Could you check a few things on this model? Use its own coordinates, in mm. Coordinates: 2 decimals unless noted, no trailing zeros. Loops run counter-clockwise (first coordinate to the right, second up) from the corner with the lowest first, then second, coordinate; pieces in that order, holes last.
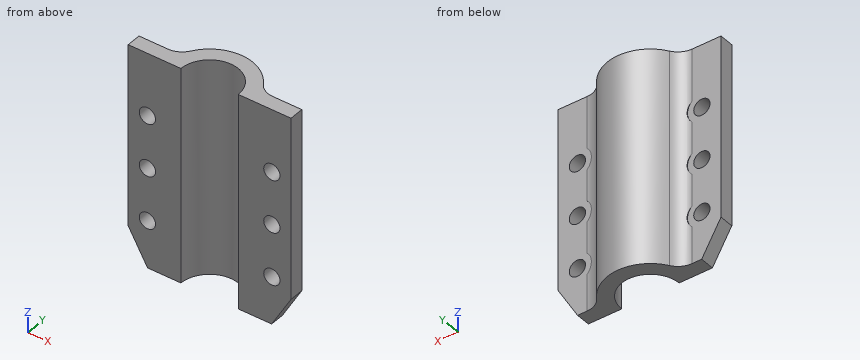
Autodesk Inventor part; units mm, degrees
ref_plane "Płaszczyzna konstrukcyjna1" through (0, 0, 50) normal (-1, 0, 0) x (0, 0, 1)
ref_plane "YZ Plane" through (0, 0, 0) normal (1, 0, 0) x (0, 1, 0)
ref_plane "XZ Plane" through (0, 0, 0) normal (0, 1, 0) x (-1, 0, 0)
sketch "Szkic1" plane through (0, 0, 0) normal (0, 0, 1) x (1, 0, 0)
  circle A0 centre (0, 0) radius 6
  circle A1 centre (0, 0) radius 9
  dimension "d0" = 12
  dimension "d1" = 18
extrude "Wyciągnięcie proste1" add sketch "Szkic1" along normal blind 50
sketch "Szkic2" plane through (0, 0, 50) normal (0, 0, 1) x (1, 0, 0)
  line L0 (-7.2, 0) -> (-20, 0)
  line L1 (-20, 0) -> (-20, 3)
  line L2 (-20, 3) -> (-7.2, 3)
  line L3 (-7.2, 3) -> (-7.2, 0)
  point P0 (0, 0)
  dimension "d4" = 3
  dimension "d5" = 7.2
  dimension "d6" = 20
extrude "Wyciągnięcie proste2" add sketch "Szkic2" against normal blind 50
ref_plane "Płaszczyzna konstrukcyjna1" through (0, 0, 50) normal (-1, 0, 0) x (0, 0, 1)
sketch "Szkic3" plane through (0, 0, 50) normal (0, 0, 1) x (1, 0, 0)
  arc A0 (-9, 0) -> (-8.4853, 3) centre (0, 0) ccw
  line L0 (-9, 0) -> (13.5216, 0)
  line L1 (13.5216, 0) -> (13.5216, -10.7801)
  line L2 (13.5216, -10.7801) -> (-9, -10.7801)
  line L3 (-9, -10.7801) -> (-9, 0)
extrude "Wyciągnięcie proste3" cut sketch "Szkic3" against normal blind 50
sketch "Szkic5" plane through (-20, 3, 50) normal (0, 1, 0) x (1, 0, 0)
  circle A0 centre (7, 13.1) radius 1.7
  circle A1 centre (7, 24.1) radius 1.7
  circle A2 centre (7, 35.1) radius 1.7
  line L0 (0, 0) -> (11.5147, 0)
  line L1 (20, -10) -> (20, 60)
  point P0 (20, 50)
  dimension "d12" = 3.4
  dimension "d13" = 3.4
  dimension "d14" = 3.4
  dimension "d16" = 13.1
  dimension "d17" = 11
  dimension "d18" = 11
  dimension "d19" = 13
  dimension "d20" = 0
  dimension "d21" = 0
extrude "Wyciągnięcie proste4" cut sketch "Szkic5" against normal blind 50
fillet "Zaokrąglenie1" radius 4 1 edges at (-8.4853, 3, 25)
mirror "Odbij1" about plane through (0, 0, 50) normal (-1, 0, 0) of "Wyciągnięcie proste2", "Wyciągnięcie proste4", "Zaokrąglenie1"
sketch "Szkic6" plane through (6, 0, 0) normal (0, -1, 0) x (1, 0, 0)
  line L0 (15.0838, 0) -> (-24.5144, 0)
  line L1 (-24.5144, 0) -> (-24.5144, 5)
  line L2 (-24.5144, 5) -> (15.0838, 5)
  line L3 (15.0838, 5) -> (15.0838, 0)
  point P0 (-6, 0)
  dimension "d28" = 5
extrude "Wyciągnięcie proste5" cut sketch "Szkic6" against normal blind 50
sketch "Szkic8" plane through (-20, 3, 50) normal (0, 1, 0) x (1, 0, 0)
  line L0 (-3.2921, -2.8939) -> (3, -2.8939)
  line L1 (3, -2.8939) -> (3, 49.96)
  line L2 (3, 49.96) -> (-3.2921, 49.96)
  line L3 (-3.2921, 49.96) -> (-3.2921, -2.8939)
  line L4 (37, 48) -> (48.6867, 48)
  line L5 (48.6867, 48) -> (48.6867, -7.6985)
  line L6 (48.6867, -7.6985) -> (37, -7.6985)
  line L7 (37, -7.6985) -> (37, 48)
  circle A0 centre (33, 35.1) radius 1.7
  circle A1 centre (7, 35.1) radius 1.7
  point P0 (20, 50)
  dimension "d32" = 4
  dimension "d33" = 4
extrude "Wyciągnięcie proste6" cut sketch "Szkic8" against normal blind 50 contours L3 L2 L1 L0 | L4 L5 L6 L7
chamfer "Faza2" distance 7 angle 30 1 edges at (17, 1.5, 5) measured on face at (17, 1, 35)
chamfer "Faza3" distance 7 angle 30 1 edges at (-17, 1.5, 5) measured on face at (-17, 1, 35)
sketch "Szkic9" plane through (-20, 3, 0.04) normal (0, 0, 1) x (1, 0, 0)
  line L0 (-2.5115, 2.374) -> (2.3445, 2.374)
  line L1 (2.3445, 2.374) -> (2.3445, -9.0767)
  line L2 (2.3445, -9.0767) -> (-2.5115, -9.0767)
  line L3 (-2.5115, -9.0767) -> (-2.5115, 2.374)
  point P0 (20, -3)
extrude "Wyciągnięcie proste7" cut sketch "Szkic9" against normal blind 50
sketch "Szkic11" plane through (-10.9545, 3, 50) normal (0, 1, 0) x (1, 0, 0)
  circle A0 centre (-2.0455, 35.1) radius 3
  circle A1 centre (-2.0455, 13.1) radius 3
  circle A2 centre (-2.0455, 24.1) radius 3
  circle A3 centre (23.9545, 35.1) radius 3
  circle A4 centre (23.9545, 24.1) radius 3
  circle A5 centre (23.9545, 13.1) radius 3
  circle A6 centre (23.9545, 35.1) radius 1.7
  circle A7 centre (23.9545, 24.1) radius 1.7
  circle A8 centre (23.9545, 13.1) radius 1.7
  circle A9 centre (-2.0455, 13.1) radius 1.7
  circle A10 centre (-2.0455, 24.1) radius 1.7
  circle A11 centre (-2.0455, 35.1) radius 1.7
  point P0 (10.9545, 50)
  dimension "d47" = 6
  dimension "d48" = 6
  dimension "d49" = 6
  dimension "d50" = 6
  dimension "d51" = 6
  dimension "d52" = 6
extrude "Wyciągnięcie proste9" cut sketch "Szkic11" along normal blind 50
properties part number "Cartesian1_X_RodCover" material "Tworzywo sztuczne ABS"
(1) Imagine slicing it at C-C, the plane x = -13.5. Write out the boundary of the cut face in (y, z).
Answers:
outline: (0, 5.94) - (3, 5.94) - (3, 13.28) - (0, 13.28) - close; (0, 16.52) - (3, 16.52) - (3, 24.28) - (0, 24.28) - close; (0, 27.52) - (3, 27.52) - (3, 35.28) - (0, 35.28) - close; (0, 38.52) - (3, 38.52) - (3, 50) - (0, 50) - close
(2) Imagine slicing it at A-A, the plane z = 14.9. Write out the boundary of the cut face in (x, y).
Answers:
outline: (-17, 0) - (-14.7, 0) - (-14.7, 3) - (-17, 3) - close; (-11.3, 0) - (-6, 0) arc R6 cw to (6, 0) - (11.3, 0) - (11.3, 3) - (10, 3) - (10, 3.12) arc R4 cw to (7.58, 4.85) arc R9 ccw to (-7.58, 4.85) arc R4 cw to (-10, 3.12) - (-10, 3) - (-11.3, 3) - close; (14.7, 0) - (17, 0) - (17, 3) - (14.7, 3) - close
(3) Imagine slicing it at D-D, the plane z = 40. Write out the boundary of the cut face in (x, y).
Answers:
outline: (-17, 0) - (-6, 0) arc R6 cw to (6, 0) - (17, 0) - (17, 3) - (10.95, 3) arc R4 cw to (7.58, 4.85) arc R9 ccw to (-7.58, 4.85) arc R4 cw to (-10.95, 3) - (-17, 3) - close
(4) For pin 1 (2.5 mm diameter, centred on x = -13, z = 14.9, fed in from +Y); pin 2 (6 mm diameter, centred on x = -7.5, z = 14.5, fed in from +Y); pin 3 (3 mm diameter, centred on x = -6.5, z = 44, fed in from +Y); pin 4 (4.5 mm diameter, centred on x = 13, z = 25.9, fed in from +Y), each with a flat end and sliding along its axis, tell me the tip position at first contact or that it passes through.
Answers:
pin 1: passes through
pin 2: stops at y = 7.79
pin 3: stops at y = 7.48
pin 4: stops at y = 3
(5) Imagine slicing it at B-B, the plane y = 1.5. Write out the boundary of the cut face in (x, z), and give its area (3 significant figures).
Answers:
outline: (-17, 12) - (-12.96, 5) - (-5.81, 5) - (-5.81, 50) - (-17, 50) - close; (5.81, 5) - (12.96, 5) - (17, 12) - (17, 50) - (5.81, 50) - close; hole circle Ø3.4 at (-13, 14.9); hole circle Ø3.4 at (-13, 25.9); hole circle Ø3.4 at (-13, 36.9); hole circle Ø3.4 at (13, 14.9); hole circle Ø3.4 at (13, 25.9); hole circle Ø3.4 at (13, 36.9)
area: 924 mm2
(6) I need wall thicknesses on probe 1 along X at (y, z) = (2, 15); probe 2 along X at (y, z) = (1.1, 36.9); probe 3 along Y at (x, z) = (-12, 21). Which ranges of each line are inside material? Lowest first, please.
Answers:
probe 1: x = -17 to -14.7, -11.3 to -5.66, 5.66 to 11.3, 14.7 to 17
probe 2: x = -17 to -14.7, -11.3 to -5.9, 5.9 to 11.3, 14.7 to 17
probe 3: y = 0 to 3
